Model file for the job. Use its own axes, mm. Coordinates: 2 decimals unless noted, no trailing zeros. Order: outer loops, then holes, each group sorted by start corner. A loop starts at its lowest first (then second) coordinate and runs counter-clockwise, first axis right, second up. Notation, with made-up numbers: M 54.5,44 L 72.5,44 A23 cw 72.5,52 Z; hole C -23,-19.5 d11. An arc over 180 degrees is marked long. Return JSON: item names as keys, results as strings.
Autodesk Inventor part; units mm, degrees
ref_plane "YZ Plane" through (0, 0, 0) normal (1, 0, 0) x (0, 1, 0)
ref_plane "XZ Plane" through (0, 0, 0) normal (0, 1, 0) x (-1, 0, 0)
ref_plane "XY Plane" through (0, 0, 0) normal (0, 0, 1) x (1, 0, 0)
sketch "Sketch1" plane through (0, 0, 0) normal (0, 0, 1) x (1, 0, 0)
  line L0 (9.9495, -14.97) -> (12.0175, -14.97)
  line L1 (9.9495, -20.042) -> (9.9495, -14.97)
  line L2 (4.9095, -20.042) -> (9.9495, -20.042)
  line L3 (4.9095, -15.47) -> (4.9095, -20.042)
  line L4 (-10.8425, -15.47) -> (4.9095, -15.47)
  line L5 (-10.8425, 10.39) -> (-10.8425, -15.47)
  line L6 (-7.5245, 10.39) -> (-10.8425, 10.39)
  line L7 (-7.5245, 30.75) -> (-7.5245, 10.39)
  line L8 (-12.0175, 30.75) -> (-7.5245, 30.75)
  line L9 (-12.0175, -25.67) -> (-12.0175, 30.75)
  line L10 (30.7975, -25.67) -> (-12.0175, -25.67)
  spline S0 degree 3 poles (31.7975, -27.4021) (31.7975, -27.1472) (31.7079, -26.8547) (31.4014, -26.2852) (31.0746, -25.9471) (30.7975, -25.67) knots 0.505532 0.505532 0.505532 0.505532 0.581995 0.581995 0.699558 0.699558 0.699558 0.699558
  line L11 (31.7975, -32.02) -> (31.7975, -27.4021)
  line L12 (33.7975, -32.02) -> (31.7975, -32.02)
  line L13 (33.7975, -32.02) -> (33.7975, -17.51)
  line L14 (12.0175, -17.51) -> (33.7975, -17.51)
  line L15 (12.0175, -14.97) -> (12.0175, -17.51)
  line L16 (4.9095, 10.39) -> (-2.5085, 10.39)
  line L17 (4.9095, 14.962) -> (4.9095, 10.39)
  line L18 (9.9495, 14.962) -> (4.9095, 14.962)
  line L19 (9.9495, 9.89) -> (9.9495, 14.962)
  line L20 (12.0175, 9.89) -> (9.9495, 9.89)
  line L21 (12.0175, 22.59) -> (12.0175, 9.89)
  line L22 (33.7975, 22.59) -> (12.0175, 22.59)
  line L23 (33.7975, 22.59) -> (33.7975, 37.1)
  line L24 (31.7975, 37.1) -> (33.7975, 37.1)
  line L25 (31.7975, 32.4821) -> (31.7975, 37.1)
  spline S1 degree 3 poles (30.7975, 30.75) (31.0746, 31.0271) (31.4014, 31.3652) (31.7079, 31.9347) (31.7975, 32.2272) (31.7975, 32.4821) knots 0 0 0 0 0.117563 0.117563 0.194026 0.194026 0.194026 0.194026
  line L26 (-2.5085, 30.75) -> (30.7975, 30.75)
  line L27 (-2.5085, 10.39) -> (-2.5085, 30.75)
  line L28 (10.0175, -25.67) -> (-0.5085, -25.67)
  line L29 (-2.5085, -23.67) -> (-2.5085, 28.75)
  line L30 (-0.5085, 30.75) -> (10.0175, 30.75)
  line L31 (12.0175, 28.75) -> (12.0175, -23.67)
  arc A0 (-2.5085, -23.67) -> (-0.5085, -25.67) centre (-0.5085, -23.67) ccw
  arc A1 (10.0175, -25.67) -> (12.0175, -23.67) centre (10.0175, -23.67) ccw
  arc A2 (-0.5085, 30.75) -> (-2.5085, 28.75) centre (-0.5085, 28.75) ccw
  arc A3 (12.0175, 28.75) -> (10.0175, 30.75) centre (10.0175, 28.75) ccw
  circle A4 centre (4.7545, -22.67) radius 1.625
  circle A5 centre (4.7545, 27.75) radius 1.625
  point P0 (0, 0)
  point P1 (12.0175, -25.67)
  dimension "d0" = 2
extrude "Extrusion1" add sketch "Sketch1" along normal blind 3 contours L1 L2 L3 L4 L29 L16 L17 L18 L19 L20 L31 L0 | L0 L15 L31 A1 L10 A0 L29 L4 L3 L2 L1 | L20 L19 L18 L17 L16 L27 A2 L26 A3 L31 L21 | A4 | A5
sketch "Sketch2" plane through (0, 0, 3) normal (0, 0, 1) x (1, 0, 0)
  line L0 (9.9495, -14.97) -> (12.0175, -14.97)
  line L1 (9.9495, -20.042) -> (9.9495, -14.97)
  line L2 (4.9095, -20.042) -> (9.9495, -20.042)
  line L3 (4.9095, -15.47) -> (4.9095, -20.042)
  line L4 (-10.8425, -15.47) -> (4.9095, -15.47)
  line L5 (-10.8425, 10.39) -> (-10.8425, -15.47)
  line L6 (-7.5245, 10.39) -> (-10.8425, 10.39)
  line L7 (-7.5245, 30.75) -> (-7.5245, 10.39)
  line L8 (-12.0175, 30.75) -> (-7.5245, 30.75)
  line L9 (-12.0175, -25.67) -> (-12.0175, 30.75)
  line L10 (30.7975, -25.67) -> (-12.0175, -25.67)
  spline S0 degree 3 poles (31.7975, -27.4021) (31.7975, -27.1472) (31.7079, -26.8547) (31.4014, -26.2852) (31.0746, -25.9471) (30.7975, -25.67) knots 0.505532 0.505532 0.505532 0.505532 0.581995 0.581995 0.699558 0.699558 0.699558 0.699558
  line L11 (31.7975, -32.02) -> (31.7975, -27.4021)
  line L12 (33.7975, -32.02) -> (31.7975, -32.02)
  line L13 (33.7975, -32.02) -> (33.7975, -17.51)
  line L14 (12.0175, -17.51) -> (33.7975, -17.51)
  line L15 (12.0175, -14.97) -> (12.0175, -17.51)
  line L16 (4.9095, 10.39) -> (-2.5085, 10.39)
  line L17 (4.9095, 14.962) -> (4.9095, 10.39)
  line L18 (9.9495, 14.962) -> (4.9095, 14.962)
  line L19 (9.9495, 9.89) -> (9.9495, 14.962)
  line L20 (12.0175, 9.89) -> (9.9495, 9.89)
  line L21 (12.0175, 22.59) -> (12.0175, 9.89)
  line L22 (33.7975, 22.59) -> (12.0175, 22.59)
  line L23 (33.7975, 22.59) -> (33.7975, 37.1)
  line L24 (31.7975, 37.1) -> (33.7975, 37.1)
  line L25 (31.7975, 32.4821) -> (31.7975, 37.1)
  spline S1 degree 3 poles (30.7975, 30.75) (31.0746, 31.0271) (31.4014, 31.3652) (31.7079, 31.9347) (31.7975, 32.2272) (31.7975, 32.4821) knots 0 0 0 0 0.117563 0.117563 0.194026 0.194026 0.194026 0.194026
  line L26 (-2.5085, 30.75) -> (30.7975, 30.75)
  line L27 (-2.5085, 10.39) -> (-2.5085, 30.75)
  line L28 (-2.5085, 28.75) -> (-2.5085, -23.67)
  arc A0 (-2.5085, -23.67) -> (-0.5085, -25.67) centre (-0.5085, -23.67) ccw
  line L29 (-0.5085, -25.67) -> (10.0175, -25.67)
  arc A1 (10.0175, -25.67) -> (12.0175, -23.67) centre (10.0175, -23.67) ccw
  line L30 (12.0175, -23.67) -> (12.0175, 28.75)
  arc A2 (12.0175, 28.75) -> (10.0175, 30.75) centre (10.0175, 28.75) ccw
  line L31 (10.0175, 30.75) -> (-0.5085, 30.75)
  arc A3 (-0.5085, 30.75) -> (-2.5085, 28.75) centre (-0.5085, 28.75) ccw
  line L32 (-0.5085, -25.67) -> (10.0175, -25.67)
  line L33 (4.7545, -25.67) -> (4.7545, -22.67)
  circle A4 centre (4.7545, -22.67) radius 1.75
  line L34 (0, 0) -> (-38.7909, 0)
  line L35 (4.7545, 30.75) -> (4.7545, 27.75)
  circle A5 centre (4.7545, 27.75) radius 1.75
  circle A6 centre (4.7545, -22.67) radius 1.625
  circle A7 centre (4.7545, 27.75) radius 1.625
  dimension "d3" = 3
  dimension "d4" = 3.5
  dimension "d5" = 3
  dimension "d6" = 3.5
extrude "Extrusion2" cut sketch "Sketch2" against normal blind 3 contours A6 | A4 | A7 | A5
properties part number "SteerServoClamp"
Item 1: Pull direction X, two halves, no side cores. Call faces 1 (the cylindrical face through (4.527, -20.935, 1.521)), 2 (the flat face through (5, 30.75, 1)), 3 (the cylindrical face through (3.46, 28.93, 1.52)), 4 (the flat face through (-2.508, 2, 1)): +X half, -X half, draft (parallel to the pull), parting line (faces both ways), or undercut.
Check result:
{"face 1": "undercut", "face 2": "draft", "face 3": "undercut", "face 4": "-X half"}
Item 2: Wall check: line 1 (Y direction, x = 4.75, z = 1.75); line 2 (X direction, y = 27.75, z = 1.75); line 3 (Y direction, x = 6, z = 1.05). Give the ranges that are in metal, low to high.
Check result:
{"line 1": "y = -25.67 to -24.42, -20.92 to 26, 29.5 to 30.75", "line 2": "x = -2.51 to 3, 6.5 to 12.02", "line 3": "y = -25.67 to -23.9, -21.44 to 26.52, 28.98 to 30.75"}
Item 3: Saw through at B-B (y = 27.75). Write the cut outline in (x, z).
Check result:
{"outline": "M -2.51,0 L 3,0 L 3,3 L -2.51,3 Z; M 6.5,0 L 12.02,0 L 12.02,3 L 6.5,3 Z"}
Item 4: Drop a flat-ended pin along its axis: pin 1 Ø3 at (x, y) = (4.75, -22.67) entering from +Z. Give the stop position or say it passes through.
Check result:
{"pin 1": "passes through"}
Item 5: Saw through at A-A (z = 2). Write the cut outline in (x, y).
Check result:
{"outline": "M -2.51,-23.67 A2 ccw -0.51,-25.67 L 10.02,-25.67 A2 ccw 12.02,-23.67 L 12.02,28.75 A2 ccw 10.02,30.75 L -0.51,30.75 A2 ccw -2.51,28.75 Z; hole C 4.75,-22.67 d3.5; hole C 4.75,27.75 d3.5"}
